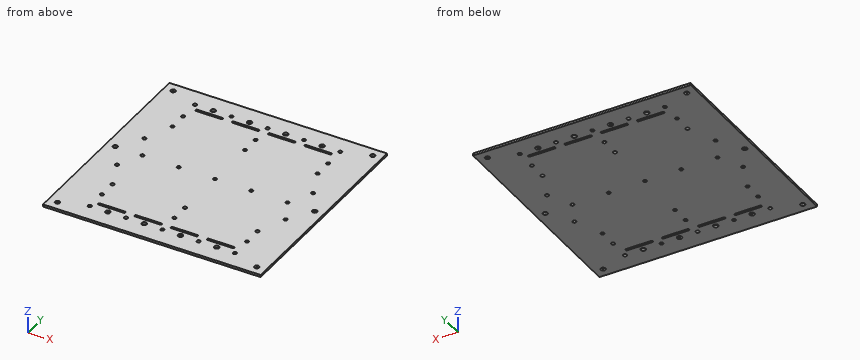
```python
from build123d import *

# Parameters (mm, degrees)
SKETCH1_W           = 304.8
SKETCH1_H           = 304.8
SKETCH1_R           = 3.3655
SKETCH1_R_2         = 2.54
SKETCH1_R_3         = 3.2639
BOSS_EXTRUDE1_DEPTH = 3.175


with BuildPart() as part:
    # Sketch1 → Boss-Extrude1 (new body)
    with BuildSketch(Plane.XY):
        Rectangle(SKETCH1_W, SKETCH1_H)
        with Locations((-76.2, 127)):
            Circle(SKETCH1_R, mode=Mode.SUBTRACT)
        with Locations((-25.4, 127)):
            Circle(SKETCH1_R, mode=Mode.SUBTRACT)
        with Locations((25.4, 127)):
            Circle(SKETCH1_R, mode=Mode.SUBTRACT)
        with Locations((76.2, 127)):
            Circle(SKETCH1_R, mode=Mode.SUBTRACT)
        with Locations((-101.6, 0)):
            Circle(SKETCH1_R_2, mode=Mode.SUBTRACT)
        with Locations((-50.8, 0)):
            Circle(SKETCH1_R_2, mode=Mode.SUBTRACT)
        Circle(SKETCH1_R_2, mode=Mode.SUBTRACT)
        with Locations((101.6, 0)):
            Circle(SKETCH1_R_2, mode=Mode.SUBTRACT)
        with Locations((50.8, 0)):
            Circle(SKETCH1_R_2, mode=Mode.SUBTRACT)
        with Locations((-50.8, 127)):
            Circle(SKETCH1_R_2, mode=Mode.SUBTRACT)
        with Locations((0, 127)):
            Circle(SKETCH1_R_2, mode=Mode.SUBTRACT)
        with Locations((50.8, 127)):
            Circle(SKETCH1_R_2, mode=Mode.SUBTRACT)
        with Locations((-101.6, 72.39)):
            Circle(SKETCH1_R_2, mode=Mode.SUBTRACT)
        with Locations((0, 72.39)):
            Circle(SKETCH1_R_2, mode=Mode.SUBTRACT)
        with Locations((101.6, 72.39)):
            Circle(SKETCH1_R_2, mode=Mode.SUBTRACT)
        with Locations((-101.6, -72.39)):
            Circle(SKETCH1_R_2, mode=Mode.SUBTRACT)
        with Locations((0, -72.39)):
            Circle(SKETCH1_R_2, mode=Mode.SUBTRACT)
        with Locations((101.6, -72.39)):
            Circle(SKETCH1_R_2, mode=Mode.SUBTRACT)
        with Locations((-76.2, -127)):
            Circle(SKETCH1_R, mode=Mode.SUBTRACT)
        with Locations((-25.4, -127)):
            Circle(SKETCH1_R, mode=Mode.SUBTRACT)
        with Locations((25.4, -127)):
            Circle(SKETCH1_R, mode=Mode.SUBTRACT)
        with Locations((76.2, -127)):
            Circle(SKETCH1_R, mode=Mode.SUBTRACT)
        with Locations((50.8, -127)):
            Circle(SKETCH1_R_2, mode=Mode.SUBTRACT)
        with Locations((0, -127)):
            Circle(SKETCH1_R_2, mode=Mode.SUBTRACT)
        with Locations((-50.8, -127)):
            Circle(SKETCH1_R_2, mode=Mode.SUBTRACT)
        with Locations((-101.6, 97.79)):
            Circle(SKETCH1_R_2, mode=Mode.SUBTRACT)
        with Locations((0, 97.79)):
            Circle(SKETCH1_R_2, mode=Mode.SUBTRACT)
        with Locations((101.6, 97.79)):
            Circle(SKETCH1_R_2, mode=Mode.SUBTRACT)
        with Locations((101.6, 127)):
            Circle(SKETCH1_R_2, mode=Mode.SUBTRACT)
        with Locations((-101.6, 127)):
            Circle(SKETCH1_R_2, mode=Mode.SUBTRACT)
        with Locations((-118.11, 33.02)):
            Circle(SKETCH1_R_2, mode=Mode.SUBTRACT)
        with Locations((-101.6, -127)):
            Circle(SKETCH1_R_2, mode=Mode.SUBTRACT)
        with Locations((101.6, -127)):
            Circle(SKETCH1_R_2, mode=Mode.SUBTRACT)
        with Locations((101.6, -97.79)):
            Circle(SKETCH1_R_2, mode=Mode.SUBTRACT)
        with Locations((0, -97.79)):
            Circle(SKETCH1_R_2, mode=Mode.SUBTRACT)
        with Locations((-101.6, -97.79)):
            Circle(SKETCH1_R_2, mode=Mode.SUBTRACT)
        with Locations((-118.11, -33.02)):
            Circle(SKETCH1_R_2, mode=Mode.SUBTRACT)
        with Locations((-139.7, 139.7)):
            Circle(SKETCH1_R_3, mode=Mode.SUBTRACT)
        with Locations((-139.7, 0)):
            Circle(SKETCH1_R_3, mode=Mode.SUBTRACT)
        with Locations((-139.7, -139.7)):
            Circle(SKETCH1_R_3, mode=Mode.SUBTRACT)
        with Locations((139.7, -139.7)):
            Circle(SKETCH1_R_3, mode=Mode.SUBTRACT)
        with Locations((139.7, 0)):
            Circle(SKETCH1_R_3, mode=Mode.SUBTRACT)
        with Locations((139.7, 139.7)):
            Circle(SKETCH1_R_3, mode=Mode.SUBTRACT)
        with Locations((118.11, 33.02)):
            Circle(SKETCH1_R_2, mode=Mode.SUBTRACT)
        with Locations((118.11, -33.02)):
            Circle(SKETCH1_R_2, mode=Mode.SUBTRACT)
        with BuildLine():
            Line((-93.6625, 119.0625), (-58.7375, 119.0625))
            ThreePointArc((-58.7375, 119.0625), (-57.15, 117.475), (-58.7375, 115.8875))
            Line((-58.7375, 115.8875), (-93.6625, 115.8875))
            ThreePointArc((-93.6625, 115.8875), (-95.25, 117.475), (-93.6625, 119.0625))
        make_face(mode=Mode.SUBTRACT)
        with BuildLine():
            Line((-7.9375, 119.0625), (-42.8625, 119.0625))
            ThreePointArc((-42.8625, 119.0625), (-44.45, 117.475), (-42.8625, 115.8875))
            Line((-42.8625, 115.8875), (-7.9375, 115.8875))
            ThreePointArc((-7.9375, 115.8875), (-6.35, 117.475), (-7.9375, 119.0625))
        make_face(mode=Mode.SUBTRACT)
        with BuildLine():
            Line((7.9375, 119.0625), (42.8625, 119.0625))
            ThreePointArc((42.8625, 119.0625), (44.45, 117.475), (42.8625, 115.8875))
            Line((42.8625, 115.8875), (7.9375, 115.8875))
            ThreePointArc((7.9375, 115.8875), (6.35, 117.475), (7.9375, 119.0625))
        make_face(mode=Mode.SUBTRACT)
        with BuildLine():
            Line((93.6625, 119.0625), (58.7375, 119.0625))
            ThreePointArc((58.7375, 119.0625), (57.15, 117.475), (58.7375, 115.8875))
            Line((58.7375, 115.8875), (93.6625, 115.8875))
            ThreePointArc((93.6625, 115.8875), (95.25, 117.475), (93.6625, 119.0625))
        make_face(mode=Mode.SUBTRACT)
        with BuildLine():
            Line((93.6625, -119.0625), (58.7375, -119.0625))
            ThreePointArc((58.7375, -119.0625), (57.15, -117.475), (58.7375, -115.8875))
            Line((58.7375, -115.8875), (93.6625, -115.8875))
            ThreePointArc((93.6625, -115.8875), (95.25, -117.475), (93.6625, -119.0625))
        make_face(mode=Mode.SUBTRACT)
        with BuildLine():
            Line((7.9375, -119.0625), (42.8625, -119.0625))
            ThreePointArc((42.8625, -119.0625), (44.45, -117.475), (42.8625, -115.8875))
            Line((42.8625, -115.8875), (7.9375, -115.8875))
            ThreePointArc((7.9375, -115.8875), (6.35, -117.475), (7.9375, -119.0625))
        make_face(mode=Mode.SUBTRACT)
        with BuildLine():
            Line((-7.9375, -119.0625), (-42.8625, -119.0625))
            ThreePointArc((-42.8625, -119.0625), (-44.45, -117.475), (-42.8625, -115.8875))
            Line((-42.8625, -115.8875), (-7.9375, -115.8875))
            ThreePointArc((-7.9375, -115.8875), (-6.35, -117.475), (-7.9375, -119.0625))
        make_face(mode=Mode.SUBTRACT)
        with BuildLine():
            Line((-93.6625, -119.0625), (-58.7375, -119.0625))
            ThreePointArc((-58.7375, -119.0625), (-57.15, -117.475), (-58.7375, -115.8875))
            Line((-58.7375, -115.8875), (-93.6625, -115.8875))
            ThreePointArc((-93.6625, -115.8875), (-95.25, -117.475), (-93.6625, -119.0625))
        make_face(mode=Mode.SUBTRACT)
    extrude(amount=BOSS_EXTRUDE1_DEPTH)


solid = part.part
```
Input: part model. Units: mm. Frame: model coordinates. Give positions to 0.01 mm unless a question says otherwise; leave off trailing zeros. Write each loop counter-clockwise with the first axis right and the second up, starting at its lowest first coordinate (ties: lowest second). Pieces come first, ordered by that corner, then holes. Notation, with made-up numbers: (-35, 62.25) - (-30, 62.25) arc R17 cw to (-30, 73.25) - close; hole circle Ø4 at (28.25, 24.25). An arc over 180 degrees is marked (long way). Write item = value, one per line. Start each with the question number.
1. Section query B-B, the plane z = 2.55. Count the separate pieces of the cut face and the enclosed holes in it, then the cut area to 3 significant figures.
2. Section query A-A, the plane x = -87. Output: boundary loops of the cut face in (y, z) (1 decimal), then the cut area to 3 significant figures.
3. Ray query, L1, parallel to Y at x = 70, z = 0.2; L2, parallel to Y at x = -50.8, z = 1.9; L3, parallel to Y at x = -76, z = 0.3. Return the intervals inside material, ascending.
Check sheet entries:
q1.separate_pieces = 1
q1.enclosed_holes = 53
q1.area = 90,800 mm2
q2.outline = (-152.4, 0) - (-119.1, 0) - (-119.1, 3.2) - (-152.4, 3.2) - close; (-115.9, 0) - (115.9, 0) - (115.9, 3.2) - (-115.9, 3.2) - close; (119.1, 0) - (152.4, 0) - (152.4, 3.2) - (119.1, 3.2) - close
q2.area = 948 mm2
q3.L1 = -152.4 to -119.06, -115.89 to 115.89, 119.06 to 152.4
q3.L2 = -152.4 to -129.54, -124.46 to -2.54, 2.54 to 124.46, 129.54 to 152.4
q3.L3 = -152.4 to -130.36, -123.64 to -119.06, -115.89 to 115.89, 119.06 to 123.64, 130.36 to 152.4
